from build123d import *

# Parameters (mm, degrees)
SKETCH1_W           = 5
SKETCH1_H           = 25
BOSS_EXTRUDE1_DEPTH = 5


with BuildPart() as part:
    # Sketch1 → Boss-Extrude1 (new body)
    with BuildSketch(Plane(origin=(0, 0, 0), x_dir=(1, 0, 0), z_dir=(0, 1, 0))):
        Polygon((-25, 28.75), (-100, 28.75), (-100, -11.25), (-25, -11.25), (-25, -18.25), (25, -18.25), (25, -11.25), (100, -11.25), (100, 28.75), (25, 28.75), (25, 48.75), (-25, 48.75), align=None)
        with Locations((92.5, 6.25)):
            Rectangle(SKETCH1_W, SKETCH1_H, mode=Mode.SUBTRACT)
        with Locations((-92.5, 6.25)):
            Rectangle(SKETCH1_W, SKETCH1_H, mode=Mode.SUBTRACT)
    extrude(amount=BOSS_EXTRUDE1_DEPTH)


solid = part.part
Source: CAD feature listing. Evaluate the final solid. Frame: model axes, mm. A direction names the side the tool comes from. Round coordinates to 2 decimals unless told otherwise and drop trailing zeros. Order: outer loops, then holes, each group sorted by start corner. A loop starts at its lowest first (then second) coordinate and runs counter-clockwise, first axis right, second up. Notation, with made-up numbers: (-11, -28) -> (41, -28) arc R31 cw to (41, -2) -> close; hole circle Ø11 at (53, -24.75). An arc over 180 degrees is marked (long way). Answer as CSV lines item,"result".
Item 1: Section A-A, the plane z = -12.5. Return loops of the section in (x, y).
A:
outline,"(-100, 0) -> (-95, 0) -> (-95, 5) -> (-100, 5) -> close; (-90, 0) -> (90, 0) -> (90, 5) -> (-90, 5) -> close; (95, 0) -> (100, 0) -> (100, 5) -> (95, 5) -> close"
Item 2: Pin query (flat end, axial travel): pin 1 Ø1.5 at (x, y) = (53, 3.5) entering from +Z; pin 2 Ø2.5 at (y, z) = (1.5, -41) entering from -X; pin 3 Ø1.5 at (x, y) = (-93, 3.5) entering from -Z; pin 4 Ø6 at (x, z) = (-58, -12) entering from -Y. Return the tip coordinate at first contact, or that it passes through.
A:
pin 1,"z = 11.25"
pin 2,"x = -25"
pin 3,"z = -28.75"
pin 4,"y = 0"
Item 3: Section B-B, the plane y = 3.2. Return loops of the section in (x, z).
A:
outline,"(-100, -28.75) -> (-25, -28.75) -> (-25, -48.75) -> (25, -48.75) -> (25, -28.75) -> (100, -28.75) -> (100, 11.25) -> (25, 11.25) -> (25, 18.25) -> (-25, 18.25) -> (-25, 11.25) -> (-100, 11.25) -> close; hole (-95, -18.75) -> (-90, -18.75) -> (-90, 6.25) -> (-95, 6.25) -> close; hole (90, -18.75) -> (95, -18.75) -> (95, 6.25) -> (90, 6.25) -> close"
Item 4: Pull-direction query (X, two-part tool) for faces 1 (the face through (-25, 2, -39)), 2 (the face through (92, 2, -18.75)), 3 (the face through (25, 2, -39)); classes: pulls with the +X half, pulls with the -X half, needs draft (parallel to the pull), parting line crosses it, or undercut.
A:
face 1,"pulls with the -X half"
face 2,"undercut"
face 3,"pulls with the +X half"
Item 5: Section D-D, the plane z = -37.5. Return loops of the section in (x, y), plus the area to 3 significant figures.
A:
outline,"(-25, 0) -> (25, 0) -> (25, 5) -> (-25, 5) -> close"
area,"250 mm²"
Item 6: Section C-C, the plane x = -74. Return loops of the section in (y, z), plus the area to 3 significant figures.
A:
outline,"(0, -28.75) -> (5, -28.75) -> (5, 11.25) -> (0, 11.25) -> close"
area,"200 mm²"
Item 7: Line query: L1, parallel to X at y = 0.5, z = -13.5; L2, parallel to Z at x = 86, y = 2.2; L3, parallel to X at y = 2.95, z = -36. Output: solid intervals per line, ascending.
A:
L1,"-100 to -95, -90 to 90, 95 to 100"
L2,"-28.75 to 11.25"
L3,"-25 to 25"
Item 8: Reachability of faces 4 (the face through (62, 2, 11.25)), 5 (the face through (-25, 2, 15)), 6 (the face through (-1, 5, -16)), 7 (the face through (63, 2, -28.75)), 8 (the face through (-93, 2, 6.25)) from +Z, -Z, +X, -X, +Y, -Y: full face, straight path, thin tool, end or side. Return the list, or none.
A:
face 4,"+Z, +X, +Y, -Y"
face 5,"+Z, -X, +Y, -Y"
face 6,"+Z, -Z, +X, -X, +Y"
face 7,"-Z, +X, +Y, -Y"
face 8,"+Y, -Y"
